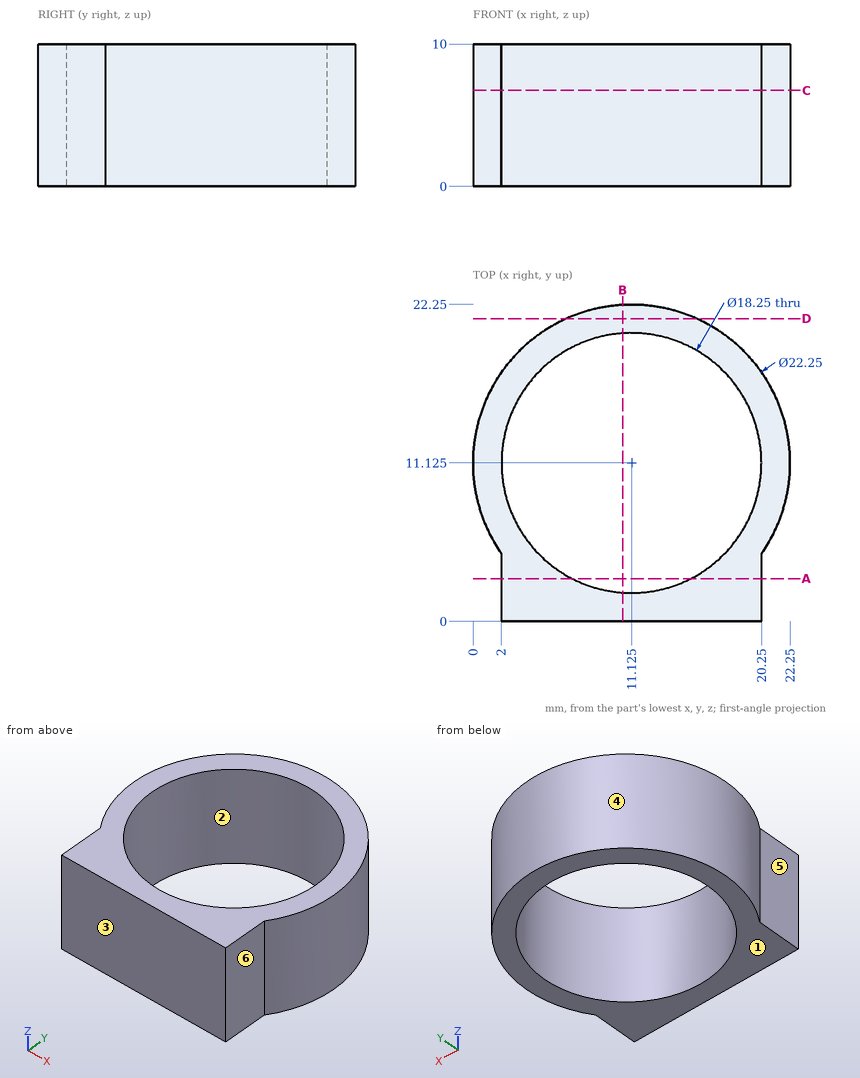
Could you check a few things on this drawing? It's one solid part, dimensions in mm from its lowest x, y, z. A direction names the side the tool comes from. Coordinates: 2 decimals unless noted, no trailing zeros. Order: outer loops, then holes, each group sorted by start corner. A loop starts at its lowest first (then second) coordinate and runs counter-clockwise, first axis right, second up. Notation, with made-up numbers: (-32, 3.25) - (-16, 3.25) arc R23 cw to (-16, 42.25) - close; hole circle Ø6 at (40.5, 19.25). An arc over 180 degrees is marked (long way). One line per question, with ' | ' between items. Start each with the question number.
1. Which directions (+Z, -Z, +X, -X, +Y, -Y) give clear straight access to the entire face, cutting with the end or side of a thin tool? Please do the marked faces 4, 5 and 6.
2. I'm going to push flat-ended pins straight in: pin 1 Ø4 at (y, z) = (5, 4.5) entering from +X; pin 2 Ø10 at (x, y) = (11, 12) entering from +Z; pin 3 Ø4 at (y, z) = (1.5, 3) entering from +X; pin 4 Ø1.5 at (y, z) = (14, 4) entering from +X. Where does each tip first touch, or does it pass through?
3. If we section it at D-D (y = 21.25): Write out the boundary of the cut face in (x, z), and give its area (3 significant figures).
4. If we section it at A-A (y = 3): Write out the boundary of the cut face in (x, z).
5. Please list where these lines run through material, in increasing order: line 1 along Y through (x, z) = (11.25, 5.75); line 2 along X through (y, z) = (5.25, 1.75); line 3 along Y through (x, z) = (9.75, 4). Write a range as [from, to].
6. If we section it at B-B (x = 10.5): Write out the boundary of the cut face in (y, z).
7. If we mould it in two halves opening along Y, with no side actions, what happens to the marked faces 1, 2 and 3? For each: released by +Y, released by -Y, zero draft, split by the parting line, or undercut.
8. If we section it at C-C (z = 6.75): Write out the boundary of the cut face in (x, y) (3 decimals), and give its area (3 significant figures).
Model answer:
1) face 4: +Z, -Z | face 5: +Z, -Z, -X, -Y | face 6: +Z, -Z, +X, -Y
2) pin 1: stops at x = 21.46 | pin 2: passes through | pin 3: stops at x = 20.25 | pin 4: stops at x = 22.05
3) outline: (6.52, 0) - (15.73, 0) - (15.73, 10) - (6.52, 10) - close | area: 92.2 mm²
4) outline: (2, 0) - (6.97, 0) - (6.97, 10) - (2, 10) - close; (15.28, 0) - (20.25, 0) - (20.25, 10) - (15.28, 10) - close
5) line 1: y = [0, 2], [20.25, 22.25] | line 2: x = [1.68, 4.14], [18.11, 20.57] | line 3: y = [0, 2.1], [20.15, 22.16]
6) outline: (0, 0) - (2.02, 0) - (2.02, 10) - (0, 10) - close; (20.23, 0) - (22.23, 0) - (22.23, 10) - (20.23, 10) - close
7) face 1: zero draft | face 2: undercut | face 3: released by -Y
8) outline: (2, 0) - (20.25, 0) - (20.25, 4.761) arc R11.125 ccw (long way) to (2, 4.761) - close; hole circle Ø18.25 at (11.125, 11.125) | area: 153 mm²
